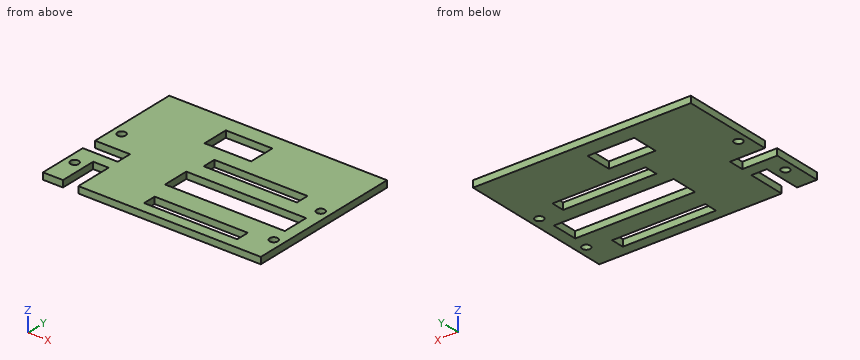
from build123d import *

# Parameters (mm, degrees)
F0_R     = 1.9812
F0_W     = 44.45
F0_H     = 6.35
F0_W_2   = 57.15
F0_H_2   = 12.7
F0_W_3   = 22.225
F1_DEPTH = 3.175


with BuildPart() as f1:
    # F0 (on Top) → F1 (new body)
    with BuildSketch(Plane.XY):
        Polygon((0, 23.7363), (0, 0), (9.51992, 0), (9.51992, 18.034), (16.88592, 18.034), (16.88592, 0), (103.886, 0), (103.886, 75.2983), (0, 75.2983), (0, 31.1023), (16.64462, 31.1023), (16.64462, 23.7363), align=None)
        with Locations((4.445, 13.2842)):
            Circle(F0_R, mode=Mode.SUBTRACT)
        with Locations((66.3575, 8.255)):
            Rectangle(F0_W, F0_H, mode=Mode.SUBTRACT)
        with Locations((99.441, 13.27912)):
            Circle(F0_R, mode=Mode.SUBTRACT)
        with Locations((69.9135, 27.432)):
            Rectangle(F0_W_2, F0_H_2, mode=Mode.SUBTRACT)
        with Locations((4.445, 41.3131)):
            Circle(F0_R, mode=Mode.SUBTRACT)
        with Locations((44.196, 61.3283)):
            Rectangle(F0_W_3, F0_H_2, mode=Mode.SUBTRACT)
        with Locations((66.1035, 44.1833)):
            Rectangle(F0_W, F0_H, mode=Mode.SUBTRACT)
        with Locations((99.441, 41.3131)):
            Circle(F0_R, mode=Mode.SUBTRACT)
    extrude(amount=F1_DEPTH)


solid = f1.part
Here's how the part is built. I have some questions about the finished solid (model axes, mm). Coordinates: 2 decimals unless noted, no trailing zeros. Write each loop counter-clockwise with the first axis right and the second up, starting at its lowest first coordinate (ties: lowest second). Pieces come first, ordered by that corner, then holes.
Item 1: I want a section at A-A on y = 7. Write out the boundary of the cut face in (x, z) (1 decimal), and give its area (3 significant figures).
Item 2: I want a section at D-D on x = 83. Write out the boundary of the cut face in (y, z) (3 decimals), and give its area (3 significant figures).
Item 3: If I drill on line 1 (Y direction, x = 58, z = 0.8); line 2 (X direction, y = 41.5, z = 1.7); line 3 (Y direction, x = 46.5, z = 0.8), over which ranges is the centre line in solid material (lowest first)?
Item 4: Will these pins go through, and if not, where does the flat tip stop? pin 1 (1.6 mm diameter, centred on y = 27, z = 2, fed in from -X); pin 2 (2.5 mm diameter, centred on x = 4.44, y = 41.31, fed in from +Z); pin 3 (1.6 mm diameter, centred on x = 14, z = 1, fed in from -Y).
Item 5: I want a section at C-C on y = 27. Write out the boundary of the cut face in (x, z) (1 decimal).
Item 6: I want a section at B-B on x = 47. Write out the boundary of the cut face in (y, z) (3 decimals), and give its area (3 significant figures).
Findings below:
1. outline: (0, 0) - (9.5, 0) - (9.5, 3.2) - (0, 3.2) - close; (16.9, 0) - (44.1, 0) - (44.1, 3.2) - (16.9, 3.2) - close; (88.6, 0) - (103.9, 0) - (103.9, 3.2) - (88.6, 3.2) - close
1. area: 165 mm2
2. outline: (0, 0) - (5.08, 0) - (5.08, 3.175) - (0, 3.175) - close; (11.43, 0) - (21.082, 0) - (21.082, 3.175) - (11.43, 3.175) - close; (33.782, 0) - (41.008, 0) - (41.008, 3.175) - (33.782, 3.175) - close; (47.358, 0) - (75.298, 0) - (75.298, 3.175) - (47.358, 3.175) - close
2. area: 158 mm2
3. line 1: y = 0 to 5.08, 11.43 to 21.08, 33.78 to 41.01, 47.36 to 75.3
3. line 2: x = 0 to 2.47, 6.42 to 43.88, 88.33 to 97.47, 101.41 to 103.89
3. line 3: y = 0 to 5.08, 11.43 to 21.08, 33.78 to 41.01, 47.36 to 54.98, 67.68 to 75.3
4. pin 1: stops at x = 16.64
4. pin 2: passes through
4. pin 3: stops at y = 18.03
5. outline: (16.6, 0) - (41.3, 0) - (41.3, 3.2) - (16.6, 3.2) - close; (98.5, 0) - (103.9, 0) - (103.9, 3.2) - (98.5, 3.2) - close
6. outline: (0, 0) - (5.08, 0) - (5.08, 3.175) - (0, 3.175) - close; (11.43, 0) - (21.082, 0) - (21.082, 3.175) - (11.43, 3.175) - close; (33.782, 0) - (41.008, 0) - (41.008, 3.175) - (33.782, 3.175) - close; (47.358, 0) - (54.978, 0) - (54.978, 3.175) - (47.358, 3.175) - close; (67.678, 0) - (75.298, 0) - (75.298, 3.175) - (67.678, 3.175) - close
6. area: 118 mm2
